Autodesk Inventor part; units mm, degrees
ref_plane "YZ Plane" through (0, 0, 0) normal (1, 0, 0) x (0, 1, 0)
ref_plane "XZ Plane" through (0, 0, 0) normal (0, 1, 0) x (-1, 0, 0)
ref_plane "XY Plane" through (0, 0, 0) normal (0, 0, 1) x (1, 0, 0)
sketch "Sketch1" plane through (0, 0, 0) normal (0, 1, 0) x (-1, 0, 0)
  line L0 (0, 0) -> (-17.78, 0)
  line L1 (-17.78, 0) -> (-17.78, -37.3888)
  line L2 (-17.78, -37.3888) -> (0, -37.3888)
  line L3 (0, -37.3888) -> (0, 0)
  circle A0 centre (-8.89, -18.6944) radius 7.62
  line L4 (0, -18.6944) -> (-17.78, -18.6944) construction
  line L5 (-8.89, -37.3888) -> (-8.89, 0) construction
  circle A1 centre (-8.89, -28.6004) radius 0.889
  circle A2 centre (-8.89, -8.7884) radius 0.889
  dimension "d0" = 37.3888
  dimension "d1" = 17.78
  dimension "d2" = 15.24
  dimension "d3" = 1.778
  dimension "d4" = 19.812
extrude "Extrusion1" add sketch "Sketch1" along normal blind 3.175
sketch "Sketch2" plane through (0, 3.175, 0) normal (0, 1, 0) x (1, 0, 0)
  line L0 (6.985, 6.8834) -> (10.795, 6.8834)
  line L1 (10.795, 6.8834) -> (10.795, 12.3482)
  line L2 (10.795, 12.3482) -> (6.985, 12.3482)
  line L3 (6.985, 12.3482) -> (6.985, 6.8834)
  circle A0 centre (8.89, 8.7884) radius 0.889 construction
  line L4 (8.89, 8.7884) -> (8.001, 8.7884) construction
  line L5 (8.89, 8.7884) -> (8.89, 9.6774) construction
  line L6 (6.985, 25.0482) -> (10.795, 25.0482)
  line L7 (10.795, 25.0482) -> (10.795, 30.513)
  line L8 (10.795, 30.513) -> (6.985, 30.513)
  line L9 (6.985, 30.513) -> (6.985, 25.0482)
  circle A1 centre (8.89, 28.6004) radius 0.889 construction
  line L10 (8.001, 28.6004) -> (8.89, 28.6004) construction
  point P0 (0, 0)
  point P1 (8.4455, 8.7884)
  point P2 (8.4455, 28.6004)
  dimension "d8" = 3.81
  dimension "d11" = 1.905
  dimension "d12" = 1.9126
  dimension "d13" = 12.7
extrude "Extrusion2" cut sketch "Sketch2" against normal blind 1.27
sketch "Sketch3" plane through (0, 3.175, 0) normal (0, 1, 0) x (1, 0, 0)
  line L0 (17.78, 37.3888) -> (0, 37.3888)
  line L1 (12.7, 37.3888) -> (5.08, 37.3888)
  line L2 (5.08, 37.3888) -> (5.08, 32.9438)
  line L3 (5.08, 32.9438) -> (12.7, 32.9438)
  line L4 (12.7, 32.9438) -> (12.7, 37.3888)
  line L5 (0, 0) -> (17.78, 0)
  line L6 (12.7, 0) -> (5.08, 0)
  line L7 (5.08, 0) -> (5.08, 4.445)
  line L8 (5.08, 4.445) -> (12.7, 4.445)
  line L9 (12.7, 4.445) -> (12.7, 0)
  line L10 (17.78, 0) -> (17.78, 37.3888) construction
  line L11 (17.78, 18.6944) -> (0, 18.6944) construction
  line L12 (0, 37.3888) -> (0, 0) construction
  circle A0 centre (8.89, 18.6944) radius 7.62 construction
  line L13 (8.89, 18.6944) -> (8.89, 11.0744) construction
  point P0 (8.89, 4.445)
  point P1 (5.08, 37.3888)
  dimension "d14" = 28.4988
  dimension "d15" = 7.62
extrude "Extrusion3" add sketch "Sketch3" against normal blind 57.15
sketch "Sketch4" plane through (17.78, 3.175, -37.3888) normal (0, 0, -1) x (-1, 0, 0)
  line L0 (12.7, -57.15) -> (5.08, -57.15)
  line L1 (12.7, -3.175) -> (12.7, -57.15)
  point P0 (17.78, -3.175)
  point P1 (8.89, -52.07)
  dimension "d18" = 5.08
  dimension "d19" = 3.81
hole "Hole1" at (8.89, -48.895, -37.3888) direction (0, 0, 1) diameter 3.175 depth 37.3888
chamfer "Chamfer1" distance 5.08 angle 70 1 edges at (17.78, 1.5875, -37.3888) measured on face at (8.89, -15.7692, -37.3888)
chamfer "Chamfer2" distance 5.08 angle 70 1 edges at (0, 1.5875, -37.3888) measured on face at (8.89, -15.7692, -37.3888)
chamfer "Chamfer3" distance 5.08 angle 70 1 edges at (17.78, 1.5875, 0) measured on face at (8.89, -15.7692, 0)
chamfer "Chamfer4" distance 5.08 angle 70 1 edges at (0, 1.5875, 0) measured on face at (8.89, -15.7692, 0)
properties part number "m500 hires mount"
For this review, take the finished solid that the model builds, in its own axes (mm). A direction names the side the tool comes from. Coordinates: 2 decimals unless noted, no trailing zeros. Loops run counter-clockwise (first coordinate to the right, second up) from the corner with the lowest first, then second, coordinate; pieces in that order, holes last. Notation, with made-up numbers: (-38, -25) - (17, -25) arc R16 ccw to (17, -2) - close; hole circle Ø4 at (65, 65). An arc over 180 degrees is marked (long way). Use one line per item in the form item = value. Start each with the question number.
1) Draft analysis for pull direction X (two halves, no side actions). For faces 1 (the face through (2.504, 1.565, -7.076)), 2 (the face through (8.41, -47.38, -2.19)), 3 (the face through (8.41, -47.38, -35.14)), 4 (the face through (12.7, -27, -35)), state which applies: released by +X, released by -X, zero draft, split by the parting line, or undercut.
2) For faces 5 (the face through (9, -27, -4.445)), 6 (the face through (9, -26, 0)), 7 (the face through (8, 1.905, -28)), list the 3-axis set-ups (+Z, -Z, +X, -X, +Y, -Y) from which the entire face can be reached by the end or side of a thin tool; tool diameter is ignored.
3) Take a section at D-D (x = 6.25). State the section outline as (y, z) points (3 decimals), plus the area to 3 significant figures.
4) To check wall thickness, follow probe 1 along Z at (x, y) = (8.89, 1.5); probe 2 along Z at (x, y) = (8.89, 2.1); probe 3 along Y at (x, z) = (8.89, -2.65) (1 decimal). State the ranges of each line that lie inside material, in increasing order. Write a range as from..to.
5) Take a section at B-B (x = 8.89). State how many separate pieces and enclosed holes the cut face has, plus the area to 3 significant figures.
6) Take a section at C-C (z = -10.5). State the section outline as (x, y) points (3 decimals), plus the area to 3 significant figures.
7) For pin 1 (8 mm diameter, centred on x = 3, y = -45.5, fed in from -Z); pin 2 (1.4 mm diameter, centred on y = 3, z = -9, fed in from -X); pin 3 (2 mm diameter, centred on y = -15.5, z = -2.5, fed in from -X); pin 4 (1.1 mm diameter, centred on x = 8.5, z = -9, fed in from +Y) (3 decimals), all flat-tipped, find the tip position at first contact; note any pin that passes through.
8) Take a section at A-A (y = -15). State the section outline as (x, z) points (3 decimals), plus the area to 3 significant figures.
From the geometry:
q1.face_1 = released by -X
q1.face_2 = undercut
q1.face_3 = undercut
q1.face_4 = released by +X
q2.face_5 = +X, -X, -Y
q2.face_6 = +Z, +X, -X, +Y, -Y
q2.face_7 = +Y
q3.outline = (-53.975, -37.389) - (3.175, -37.389) - (3.175, -25.842) - (0, -25.842) - (0, -32.944) - (-53.975, -32.944) - close; (-53.975, -4.445) - (0, -4.445) - (0, -11.546) - (3.175, -11.546) - (3.175, 0) - (-53.975, 0) - close
q3.area = 553 mm2
q4.probe_1 = -37.39..-29.49, -27.71..-26.31, -11.07..-9.68, -7.9..0
q4.probe_2 = -37.39..-30.51, -6.88..0
q4.probe_3 = -54..-50.5, -47.3..3.2
q5.separate_pieces = 6
q5.enclosed_holes = 0
q5.area = 505 mm2
q6.outline = (1.258, 0) - (16.522, 0) - (16.522, 3.175) - (10.795, 3.175) - (10.795, 1.905) - (6.985, 1.905) - (6.985, 3.175) - (1.258, 3.175) - close
q6.area = 43.6 mm2
q7.pin_1 = -37.39
q7.pin_2 = 1.55
q7.pin_3 = 5.08
q7.pin_4 = 1.905
q8.outline = (5.08, -37.389) - (12.7, -37.389) - (12.7, -32.944) - (5.08, -32.944) - close; (5.08, -4.445) - (12.7, -4.445) - (12.7, 0) - (5.08, 0) - close
q8.area = 67.7 mm2
